```python
from build123d import *

# Parameters (mm, degrees)
SKETCH1_R           = 2.5
BOSS_EXTRUDE1_DEPTH = 154
SKETCH2_R           = 3.5
BOSS_EXTRUDE2_DEPTH = 2
BOSS_EXTRUDE3_START = -2
SKETCH3_R           = 3.5
BOSS_EXTRUDE3_DEPTH = 2


with BuildPart() as part:
    # Sketch1 → Boss-Extrude1 (new body)
    with BuildSketch(Plane(origin=(0, 0, 0), x_dir=(1, 0, 0), z_dir=(0, 1, 0))):
        with Locations(Location((0, 0, 0), (0, 0, 270))):
            Circle(SKETCH1_R)
    extrude(amount=BOSS_EXTRUDE1_DEPTH)

    # Sketch2 → Boss-Extrude2 (add)
    with BuildSketch(Plane.XZ):
        with Locations(Location((0, 0, 0), (0, 0, 270))):
            Circle(SKETCH2_R)
    extrude(amount=-BOSS_EXTRUDE2_DEPTH)

    # Sketch3 → Boss-Extrude3 (add)
    with BuildSketch(Plane(origin=(0, 154, 0), x_dir=(1, 0, 0), z_dir=(0, 1, 0)).offset(BOSS_EXTRUDE3_START)):
        with Locations(Location((0, 0, 0), (0, 0, 90))):
            Circle(SKETCH3_R)
    extrude(amount=BOSS_EXTRUDE3_DEPTH)


solid = part.part
```
Verification items for the finished model (mm, model axes). A direction names the side the tool comes from. Give positions to 0.01 mm unless a question says otherwise; leave off trailing zeros. Loops run counter-clockwise (first coordinate to the right, second up) from the corner with the lowest first, then second, coordinate; pieces in that order, holes last.
1. Section check A-A, the plane z = 0. Enter the section's corners in (x, y), then the cut area to 3 significant figures.
2. Thickness scan on line 1 (Y direction, x = -2.5, z = -1.25); line 2 (X direction, y = 70, z = 0); line 3 (Z direction, x = 0.25, y = 140). Record the ranges inside material, lowest first.
3. Section check B-B, the plane x = 0. Enter the section's corners in (y, z).
4. Go/stop test with flat-tipped pins: pin 1 Ø2 at (x, y) = (1, 43) entering from +Z; pin 2 Ø3 at (x, y) = (1, 58) entering from -Z. Record where each tip stops, or that it passes through.
5. Mould release check, pull along Y, two halves, no side actions. Record for faces 3 (the flat face through (0, 0, 0)), 4 (the cylindrical face through (-2.44, 75.95, -0.54)), 5 (the cylindrical face through (3.417, 152.986, 0.759)), 6 (the flat face through (2, 152, -2)): released by +Y, released by -Y, zero draft, split by the parting line, or undercut.
6. Set-up check for faces 1 (the flat face through (-2, 2, -2)), 2 (the flat face through (0, 154, 0)): record each of +Z, -Z, +X, -X, +Y, -Y from which the full face is reachable in a straight line by a thin tool's end or side.
7. Section check C-C, the plane y = 60.5. Enter the section's corners in (x, z).
Geometry says:
1. outline: (-3.5, 0) - (3.5, 0) - (3.5, 2) - (2.5, 2) - (2.5, 152) - (3.5, 152) - (3.5, 154) - (-3.5, 154) - (-3.5, 152) - (-2.5, 152) - (-2.5, 2) - (-3.5, 2) - close
1. area: 778 mm2
2. line 1: y = 0 to 2, 152 to 154
2. line 2: x = -2.5 to 2.5
2. line 3: z = -2.49 to 2.49
3. outline: (0, -3.5) - (2, -3.5) - (2, -2.5) - (152, -2.5) - (152, -3.5) - (154, -3.5) - (154, 3.5) - (152, 3.5) - (152, 2.5) - (2, 2.5) - (2, 3.5) - (0, 3.5) - close
4. pin 1: stops at z = 2.5
4. pin 2: stops at z = -2.5
5. face 3: released by -Y
5. face 4: undercut
5. face 5: zero draft
5. face 6: undercut
6. face 1: none
6. face 2: +Z, -Z, +X, -X, +Y
7. outline: circle Ø5 at (0, 0)
